from build123d import *

# Parameters (mm, degrees)
F1_DEPTH = 67
F2_R     = 10
F3_SIZE  = 5


with BuildPart() as f1:
    # F0 (on Front) → F1 (new body)
    with BuildSketch(Plane.XZ):
        Polygon((66, 66), (0, 66), (0, 0), (162.102426, 0), (64.806874, 218.153241), (-1.859792, 218.153241), align=None)
    extrude(amount=F1_DEPTH)

    # F2
    f2_edges = [f1.edges().sort_by_distance(p)[0] for p in [
        (162.102426, -33.5, 0),
    ]]
    fillet(f2_edges, radius=F2_R)

    # F3
    f3_edges = [f1.edges().sort_by_distance(p)[0] for p in [
        (110.316348, -67, 116.113229),
        (110.316348, 0, 116.113229),
        (32.070104, -67, 142.07662),
        (32.070104, 0, 142.07662),
        (33, 0, 66),
        (33, -67, 66),
    ]]
    chamfer(f3_edges, length=F3_SIZE)


solid = f1.part
The listing builds one solid part. Answer for the finished solid, in the listing's coordinates (mm). A direction names the side the tool comes from. Coordinates: 2 decimals unless noted, no trailing zeros. Write each loop counter-clockwise with the first axis right and the second up, starting at its lowest first coordinate (ties: lowest second). Pieces come first, ordered by that corner, then holes. Notation, with made-up numbers: M 46,-18.75 L 86,-18.75 A30 cw 86,16.25 Z; hole C -24,62.5 d3. An arc over 180 degrees is marked long. Write each question's results on one line, items separated by ' | '.
Item 1: The part is cut by section B-B on x = 20.5. Determine the outline of the cut face in (y, z).
Answer below:
outline: M -67,5 L -62,0 L -5,0 L 0,5 L 0,61 L -5,66 L -62,66 L -67,61 Z; M -67,180.29 L -62,168.02 L -5,168.02 L 0,180.29 L 0,218.15 L -67,218.15 Z
Item 2: For a pull along Z with two mould halves and no side action, classify faces 1 (the face through (0, -33, 33)), 2 (the face through (35.394, -64.465, 140.677)), 3 (the face through (72, -33, 0)) as released by +Z, released by -Z, zero draft, split by the parting line, or undercut.
Answer below:
face 1: zero draft | face 2: undercut | face 3: released by -Z
Item 3: Given P1, Ø8, axis at x = 101, y = -32, coming from the +Z side; P2, Ø5, axis at y = -53, z = 124, coming from the +X side; P3, Ø5, axis at y = -52.5, z = 48, coming from the +X side, each flat-ended and moving along its own axis, determine where each tip first touches the part or whether it passes through.
Answer below:
P1: z = 145.97 | P2: x = 107.91 | P3: x = 141.81
Item 4: The part is cut by section C-C on z = 188. Determine the outline of the cut face in (x, y).
Answer below:
outline: M 11.59,-62 L 17.06,-67 L 72.78,-67 L 78.26,-62 L 78.26,-5 L 72.78,0 L 17.06,0 L 11.59,-5 Z
Item 5: The part is cut by section A-A on y = -28.5. Determine the outline of the cut face in (x, z).
Answer below:
outline: M -1.86,218.15 L 66,66 L 0,66 L 0,0 L 146.69,0 A10 ccw 155.83,14.07 L 64.81,218.15 Z
Item 6: Consider probe 1 along Z at (x, y) = (33, -17); probe 2 along X at (y, z) = (-20.5, 147.5); probe 3 along Z at (x, y) = (51.5, -61). Determine where each line is inside the solid, lowest interval first. Write a range as [from, to].
Answer below:
probe 1: [0, 66], [139.99, 218.15] | probe 2: [29.65, 96.32] | probe 3: [0, 66], [98.51, 218.15]
Item 7: Which of the six approach directions +Z, -Z, +X, -X, +Y, -Y give full straight-line access (tool end or side, diameter ignored) to faces 4 (the face through (37, -64, 64)), 5 (the face through (108.25, -64.47, 114.68)), 6 (the face through (72, -3, 2)), 7 (the face through (31.595, -33.101, 143.142)), 8 (the face through (37, -3, 64))?
Answer below:
face 4: -X, -Y | face 5: +Z, +X, -Y | face 6: -Z, +X, -X, +Y | face 7: -X, +Y, -Y | face 8: -X, +Y
Item 8: The part is cut by section D-D on x = 71. Determine the outline of the cut face in (y, z), and give its area (3 significant figures).
Answer below:
outline: M -67,5 L -62,0 L -5,0 L 0,5 L 0,61 L -1.76,62.76 L 0,67.06 L 0,191.99 L -5,204.27 L -62,204.27 L -67,191.99 L -67,67.06 L -65.24,62.76 L -67,61 Z | area: 13,600 mm2
